Design review of the part built by this model. Coordinates are the model's own, in mm. A direction names the side the tool comes from. Round coordinates to 2 decimals unless told otherwise and drop trailing zeros. Order: outer loops, then holes, each group sorted by start corner. A loop starts at its lowest first (then second) coordinate and runs counter-clockwise, first axis right, second up.
from build123d import *

# Parameters (mm, degrees)
SKETCH1_R           = 2.25
BOSS_EXTRUDE1_DEPTH = 5
SKETCH2_W           = 7
SKETCH2_H           = 9
BOSS_EXTRUDE2_DEPTH = 20
SKETCH4_W           = 9
SKETCH4_H           = 9
BOSS_EXTRUDE4_DEPTH = 20
SKETCH5_R           = 2.5
CUT_EXTRUDE1_DEPTH  = 25
FILLET1_R           = 5
FILLET2_R           = 5


with BuildPart() as part:
    # Sketch1 → Boss-Extrude1 (new body)
    with BuildSketch(Plane.XY):
        with BuildLine():
            ThreePointArc((4.5, 10), (0, 14.5), (-4.5, 10))
            Line((-4.5, 10), (-4.5, -10))
            ThreePointArc((-4.5, -10), (0, -14.5), (4.5, -10))
            Line((4.5, -10), (4.5, 10))
        make_face()
        with Locations((0, 10)):
            Circle(SKETCH1_R, mode=Mode.SUBTRACT)
        with Locations((0, -10)):
            Circle(SKETCH1_R, mode=Mode.SUBTRACT)
    extrude(amount=BOSS_EXTRUDE1_DEPTH)

    # Sketch2 → Boss-Extrude2 (add)
    with BuildSketch(Plane.XY.offset(5)):
        Rectangle(SKETCH2_W, SKETCH2_H)
    extrude(amount=BOSS_EXTRUDE2_DEPTH)

    # Sketch4 → Boss-Extrude4 (add)
    with BuildSketch(Plane(origin=(3.5, 0, 0), x_dir=(0, 0, -1), z_dir=(1, 0, 0))):
        with Locations((-20.5, 0)):
            Rectangle(SKETCH4_W, SKETCH4_H)
    extrude(amount=BOSS_EXTRUDE4_DEPTH)

    # Sketch5 → Cut-Extrude1 (cut)
    with BuildSketch(Plane(origin=(23.5, 0, 0), x_dir=(0, 0, -1), z_dir=(1, 0, 0))):
        with Locations((-20.5, 0)):
            Circle(SKETCH5_R)
    extrude(amount=-CUT_EXTRUDE1_DEPTH, mode=Mode.SUBTRACT)

    # Fillet1
    fillet1_edges = [part.edges().sort_by_distance(p)[0] for p in [
        (3.5, 0, 16),
    ]]
    fillet(fillet1_edges, radius=FILLET1_R)

    # Fillet2
    fillet2_edges = [part.edges().sort_by_distance(p)[0] for p in [
        (-3.5, 0, 25),
    ]]
    fillet(fillet2_edges, radius=FILLET2_R)


solid = part.part
1) Take a section at A-A on x = 0. Give the boundary of the cut face in (y, z), plus the area to 3 significant figures.
Results:
outline: (-14.5, 0) - (-12.25, 0) - (-12.25, 5) - (-14.5, 5) - close; (-7.75, 0) - (7.75, 0) - (7.75, 5) - (4.5, 5) - (4.5, 24.77) - (-4.5, 24.77) - (-4.5, 5) - (-7.75, 5) - close; (12.25, 0) - (14.5, 0) - (14.5, 5) - (12.25, 5) - close; hole circle Ø5 at (0, 20.5)
area: 258 mm2
2) Clearance check with flat-ended pins moving along their axes: P1, Ø1, axis at x = 9, y = 6.5, coming from the -Z side; P2, Ø10, axis at x = 9.5, z = 16.5, coming from the +Y side; P3, Ø10, axis at x = 4.5, z = 17.5, coming from the -Y side; P4, Ø3, axis at y = 2, z = 19.5, coming from the -X side. State where each tip first meets the part, or that it passes through.
Results:
P1: passes through
P2: stops at y = 4.5
P3: stops at y = -4.5
P4: stops at x = -3.5
3) Take a section at D-D on z = 18.5. Give the boundary of the cut face in (x, y), plus the area to 3 significant figures.
Results:
outline: (-3.5, -4.5) - (23.5, -4.5) - (23.5, -1.5) - (-1.5, -1.5) - (-1.5, 1.5) - (23.5, 1.5) - (23.5, 4.5) - (-3.5, 4.5) - close
area: 168 mm2
4) To check wall thickness, follow line 1 along Y through (x, z) = (0, 2.75); line 2 along Y through (x, z) = (14.5, 20.5); line 3 along X through (y, z) = (0.75, 3). State the ranges of each line that lie inside material, in increasing order.
Results:
line 1: y = -14.5 to -12.25, -7.75 to 7.75, 12.25 to 14.5
line 2: y = -4.5 to -2.5, 2.5 to 4.5
line 3: x = -4.5 to 4.5
5) Take a section at B-B on z = 3.25. Give the boundary of the cut face in (x, y).
Results:
outline: (-4.5, -10) arc R4.5 ccw to (4.5, -10) - (4.5, 10) arc R4.5 ccw to (-4.5, 10) - close; hole circle Ø4.5 at (0, -10); hole circle Ø4.5 at (0, 10)
6) For faces 1 (the face through (-3.5, 0, 12)), 2 (the face through (7, 4.5, 17)), 3 (the face through (16, 0, 16)), list the 3-axis set-ups (+Z, -Z, +X, -X, +Y, -Y) from which the entire face can be reached by the end or side of a thin tool; tool diameter is ignored.
Results:
face 1: +Z, -X, +Y, -Y
face 2: +Z, +X, -X, +Y
face 3: -Z, +X, +Y, -Y
7) The part is to be moulded in two halves that separate along X. For faces 4 (the face through (1.21, 11.897, 2.465)), 5 (the face through (0.1, 14.5, 2.5)), 6 (the face through (3.5, 0, 8)), say which applies: released by +X, released by -X, zero draft, split by the parting line, or undercut.
Results:
face 4: undercut
face 5: split by the parting line
face 6: released by +X
8) Take a section at C-C on x = 15.25. Give the boundary of the cut face in (y, z).
Results:
outline: (-4.5, 16) - (4.5, 16) - (4.5, 25) - (-4.5, 25) - close; hole circle Ø5 at (0, 20.5)
